The listing builds one solid part. Answer for the finished solid, in the listing's coordinates (mm). A direction names the side the tool comes from. Give positions to 0.01 mm unless a question says otherwise; leave off trailing zeros. Loops run counter-clockwise (first coordinate to the right, second up) from the corner with the lowest first, then second, coordinate; pieces in that order, holes last. Notation, with made-up numbers: M 75.25,-14 L 99.25,-14 A11 ccw 99.25,-5 Z; hole C -25.5,-20 d4. An arc over 180 degrees is marked long. One line per item, written item: value. Start each with the question number.
Q1. A cutting plane is placed at B-B, the plane z = 0. Determine the outline of the cut face in (x, y), and give its area (3 significant figures).
Q2. Consider L1, parallel to X at y = 4, z = -10; L2, parallel to X at y = 21.5, z = 0; L3, parallel to Y at x = 3, z = 1. Determine where each line is inside the solid, lowest interval first.
Q3. The mould has two halves that part along Z. Classify faces 4 (the cylindrical face through (8.514, 2.465, 7.375)), 5 (the cylindrical face through (20.316, 19.426, -6.398)), 6 (the flat face through (-11.1, 6.822, -17.5)): +Z half, -Z half, draft (parallel to the pull), parting line (faces both ways), or undercut.
Q4. Flat-ended cylindrical pins translate along their axes: pin 1 (3 mm diameter, centred on x = 12, z = 13.5, fed in from +Y); pin 2 (8 mm diameter, centred on x = 7.5, y = 17, fed in from +Z); pin 3 (13 mm diameter, centred on x = -7.5, z = 3.5, fed in from -Y); pin 4 (2.5 mm diameter, centred on x = 8.84, z = 8.84, fed in from -Y). Find the tip coordinate at first contact, or state that the pin passes through.
Q5. A cutting plane is placed at A-A, the plane x = 0. Determine the outline of the cut face in (y, z).
Q6. For faces 1 (the flat face through (9, 5, -9)), 2 (the flat face through (0, 36, 3)), 3 (the flat face through (11.1, 7.831, -17.5)), determine the directions among +Z, -Z, +X, -X, +Y, -Y from which every point of the face is accessible in a straight line to the end or side of a thin tool.
Q7. A cutting plane is placed at C-C, the plane y = 16.5. Determine the outline of the cut face in (x, z).
Q8. A cutting plane is placed at D-D, the plane y = 3. Determine the outline of the cut face in (x, z), and give its area (3 significant figures).
from build123d import *

# Parameters (mm, degrees)
SKETCH2_R          = 1.5
CUT_EXTRUDE1_DEPTH = 5


with BuildPart() as part:
    # Sketch1 → Revolve1 (revolve)
    with BuildSketch(Plane.XY):
        Polygon((8, 0), (16, 0), (20.8, 4.8), (21.3, 4.8), (21.3, 6.821980551), (20.529759762, 6.821980551), (20.529759762, 7.830949193), (21.3, 7.830949193), (21.3, 30.7), (16, 36), (2.5, 36), (2.5, 1), (8, 1), align=None)
    revolve(axis=Axis((0, 0, 0), (0, 1, 0)))

    # Sketch2 → Cut-Extrude1 (cut)
    with BuildSketch(Plane.XZ):
        with Locations((-8.838834765, 8.838834765)):
            Circle(SKETCH2_R)
        with Locations((8.838834765, 8.838834765)):
            Circle(SKETCH2_R)
        with Locations((8.838834765, -8.838834765)):
            Circle(SKETCH2_R)
        with Locations((-8.838834765, -8.838834765)):
            Circle(SKETCH2_R)
    extrude(amount=-CUT_EXTRUDE1_DEPTH, mode=Mode.SUBTRACT)


solid = part.part
Answer block:
1. outline: M -21.3,4.8 L -20.8,4.8 L -16,0 L -8,0 L -8,1 L -2.5,1 L -2.5,36 L -16,36 L -21.3,30.7 L -21.3,7.83 L -20.53,7.83 L -20.53,6.82 L -21.3,6.82 Z; M 2.5,1 L 8,1 L 8,0 L 16,0 L 20.8,4.8 L 21.3,4.8 L 21.3,6.82 L 20.53,6.82 L 20.53,7.83 L 21.3,7.83 L 21.3,30.7 L 16,36 L 2.5,36 Z
1. area: 1,290 mm^2
2. L1: -17.32 to -9.79, -7.89 to 7.89, 9.79 to 17.32
2. L2: -21.3 to -2.5, 2.5 to 21.3
2. L3: 1 to 36
3. face 4: undercut
3. face 5: parting line
3. face 6: draft
4. pin 1: y = 35.44
4. pin 2: z = 21.01
4. pin 3: y = 0
4. pin 4: y = 5
5. outline: M 0,-16 L 4.8,-20.8 L 4.8,-21.3 L 6.82,-21.3 L 6.82,-20.53 L 7.83,-20.53 L 7.83,-21.3 L 30.7,-21.3 L 36,-16 L 36,-2.5 L 1,-2.5 L 1,-8 L 0,-8 Z; M 0,8 L 1,8 L 1,2.5 L 36,2.5 L 36,16 L 30.7,21.3 L 7.83,21.3 L 7.83,20.53 L 6.82,20.53 L 6.82,21.3 L 4.8,21.3 L 4.8,20.8 L 0,16 Z
6. face 1: -Y
6. face 2: +Z, -Z, +X, -X, +Y
6. face 3: none
7. outline: C 0,0 d42.6; hole C 0,0 d5
8. outline: C 0,0 d38; hole C -8.84,-8.84 d3; hole C -8.84,8.84 d3; hole C 0,0 d5; hole C 8.84,-8.84 d3; hole C 8.84,8.84 d3
8. area: 1,090 mm^2
